from build123d import *

# Parameters (mm, degrees)
F0_W     = 76.2
F0_H     = 508
F0_R     = 19.05
F1_DEPTH = 76.2


with BuildPart() as f1:
    # F0 (on Front) → F1 (new body)
    with BuildSketch(Plane.XZ):
        with Locations((-111.027259, 146.427681)):
            Rectangle(F0_W, F0_H)
        with Locations((-111.027259, -77.092319)):
            Circle(F0_R, mode=Mode.SUBTRACT)
        with Locations((-111.027259, -31.372319)):
            Circle(F0_R, mode=Mode.SUBTRACT)
        with Locations((-111.027259, 14.347681)):
            Circle(F0_R, mode=Mode.SUBTRACT)
        with Locations((-111.027259, 58.797681)):
            Circle(F0_R, mode=Mode.SUBTRACT)
        with Locations((-111.027259, 103.247681)):
            Circle(F0_R, mode=Mode.SUBTRACT)
        with Locations((-111.027259, 146.427681)):
            Circle(F0_R, mode=Mode.SUBTRACT)
        with Locations((-111.027259, 189.607681)):
            Circle(F0_R, mode=Mode.SUBTRACT)
        with Locations((-111.027259, 234.057681)):
            Circle(F0_R, mode=Mode.SUBTRACT)
        with Locations((-111.027259, 278.507681)):
            Circle(F0_R, mode=Mode.SUBTRACT)
        with Locations((-111.027259, 324.227681)):
            Circle(F0_R, mode=Mode.SUBTRACT)
        with Locations((-111.027259, 369.947681)):
            Circle(F0_R, mode=Mode.SUBTRACT)
    extrude(amount=F1_DEPTH)


solid = f1.part
CAD build for the part. Positions are in the model's coordinates, mm. Coordinates: 2 decimals unless noted, no trailing zeros. Order: outer loops, then holes, each group sorted by start corner. A loop starts at its lowest first (then second) coordinate and runs counter-clockwise, first axis right, second up.
Item 1: Band-saw the part on D-D on z = -68. List the corners of the cut face in (x, y), plus the area to 3 significant figures.
Check sheet entries:
outline: (-149.13, -76.2) - (-127.77, -76.2) - (-127.77, 0) - (-149.13, 0) - close; (-94.29, -76.2) - (-72.93, -76.2) - (-72.93, 0) - (-94.29, 0) - close
area: 3,260 mm2
Item 2: Band-saw the part on A-A on z = 141. List the corners of the cut face in (x, y).
Check sheet entries:
outline: (-149.13, -76.2) - (-129.29, -76.2) - (-129.29, 0) - (-149.13, 0) - close; (-92.77, -76.2) - (-72.93, -76.2) - (-72.93, 0) - (-92.77, 0) - close
Item 3: Band-saw the part on B-B on y = -5. Give the number of separate pieces and of enclosed holes in the cut face, plus the area to 3 significant figures.
Check sheet entries:
separate pieces: 1
enclosed holes: 11
area: 26,200 mm2
Item 4: Pin check, flat tip, straight feed: pin 1 Ø23 at (x, z) = (-111.03, 103.25) entering from -Y. Stop position of the tip, or through.
Check sheet entries:
pin 1: passes through
Item 5: Drill centre lines: L1, parallel to X at y = -27, z = 324; L2, parallel to X at y = -65.5, z = 264. Where is each one in solid material? Low to high.
Check sheet entries:
L1: x = -149.13 to -130.08, -91.98 to -72.93
L2: x = -149.13 to -123.37, -98.68 to -72.93
